Read the model definition and answer for the solid it produces. Units are mm, in the model's axes. A direction names the side the tool comes from. Coordinates: 2 decimals unless noted, no trailing zeros. Write each loop counter-clockwise with the first axis right and the second up, starting at its lowest first coordinate (ties: lowest second). Pieces come first, ordered by that corner, then holes. Notation, with made-up numbers: M 39.5,-35 L 66.5,-35 A10 ccw 66.5,-23 Z; hole C -4,-25.75 d8. An arc over 180 degrees is marked long. Write item = value, one per line.
from build123d import *

# Parameters (mm, degrees)
P_IDAT_VYSUNUT_M5_DEPTH = 1.6
P_IDAT_VYSUNUT_M6_DEPTH = 1
P_IDAT_VYSUNUT_M7_DEPTH = 3
ZKOSEN_1_SIZE           = 3
ZKOSEN_1_SIZE_2         = 1.398922974


with BuildPart() as part:
    # Skica1 → Přidat vysunutím5 (new body)
    with BuildSketch(Plane.XY):
        Polygon((0, 0), (0, 20), (-12.412784718, 31.615626352), (-23, 25), (-23, 0), align=None)
    extrude(amount=P_IDAT_VYSUNUT_M5_DEPTH)

    # Skica2 → Přidat vysunutím6 (add)
    with BuildSketch(Plane.XY.offset(1.6)):
        with BuildLine():
            Line((-3.705128205, 4.115384615), (-3.705128205, 2))
            Line((-3.705128205, 2), (-10.897435897, 2))
            add(Edge.make_bspline(
                [(-10.897435897, 2), (-10.87308441, 2.180790308), (-10.824395089, 2.542269551), (-10.673865117, 3.070299742), (-10.472959166, 3.585566992), (-10.254913916, 4.004869463), (-10.038043764, 4.342393523), (-9.841277463, 4.618963346), (-9.60654249, 4.913221767), (-9.337245105, 5.227544267), (-9.034873554, 5.562913411), (-8.697171951, 5.918082368), (-8.322529407, 6.291350846), (-8.058961705, 6.54481851), (-7.922676282, 6.67588141)],
                knots=[0, 0, 0, 0, 1.156289446, 2.311930546, 3.473459201, 4.661751613, 5.303057008, 6.018253237, 6.81459331, 7.690699809, 8.644447906, 9.679642995, 10.800191253, 12, 12, 12, 12], degree=3))
            add(Edge.make_bspline(
                [(-7.922676282, 6.67588141), (-7.813918956, 6.780862005), (-7.606877039, 6.980714138), (-7.312048947, 7.266894293), (-7.052864674, 7.529975199), (-6.823905036, 7.763139303), (-6.630459323, 7.972323552), (-6.469982936, 8.154242742), (-6.34044346, 8.309637702), (-6.270284768, 8.408220362), (-6.239182692, 8.451923077)],
                knots=[0, 0, 0, 0, 1.480720495, 2.818855715, 4.024636094, 5.098235712, 6.019786162, 6.815086302, 7.474715479, 8, 8, 8, 8], degree=3))
            add(Edge.make_bspline(
                [(-6.239182692, 8.451923077), (-6.175493233, 8.557718073), (-6.052643645, 8.761784362), (-5.91792888, 9.082682292), (-5.837068057, 9.403513936), (-5.825971765, 9.617891805), (-5.820512821, 9.723357372)],
                knots=[0, 0, 0, 0, 1.0911822, 2.104764037, 3.067617678, 4, 4, 4, 4], degree=3))
            add(Edge.make_bspline(
                [(-5.820512821, 9.723357372), (-5.824474653, 9.833108474), (-5.831970132, 10.040748999), (-5.894821019, 10.333768175), (-6.006276867, 10.585659667), (-6.15973106, 10.797196661), (-6.353774193, 10.962935085), (-6.580616259, 11.085399693), (-6.843577862, 11.153106661), (-7.028402789, 11.16201224), (-7.125, 11.166666667)],
                knots=[0, 0, 0, 0, 1.193122327, 2.257294386, 3.237245624, 4.168877528, 5.075331632, 5.990371598, 6.949684428, 8, 8, 8, 8], degree=3))
            add(Edge.make_bspline(
                [(-7.125, 11.166666667), (-7.220944609, 11.16231978), (-7.406288878, 11.153922533), (-7.669703299, 11.080565334), (-7.900142302, 10.953576306), (-8.06436539, 10.808860058), (-8.175305876, 10.668134018), (-8.250896853, 10.545500545), (-8.316050374, 10.406151312), (-8.37378183, 10.251655158), (-8.419383153, 10.080242168), (-8.456107626, 9.893217825), (-8.485702239, 9.689575671), (-8.495113848, 9.547907653), (-8.5, 9.474358974)],
                knots=[0, 0, 0, 0, 1.402788338, 2.709884207, 3.961032948, 5.225417836, 5.883680772, 6.578928686, 7.329201998, 8.132101139, 8.990263233, 9.922304639, 10.921339128, 12, 12, 12, 12], degree=3))
            Line((-8.5, 9.474358974), (-10.615384615, 9.681490385))
            add(Edge.make_bspline(
                [(-10.615384615, 9.681490385), (-10.598377251, 9.824305509), (-10.565402688, 10.101201217), (-10.483114114, 10.498918926), (-10.378898684, 10.865831465), (-10.247788098, 11.201257911), (-10.095201314, 11.507331251), (-9.913355139, 11.779458664), (-9.708603468, 12.020654551), (-9.480769352, 12.230790543), (-9.231301205, 12.410535137), (-8.969529148, 12.57098477), (-8.690337423, 12.702604473), (-8.396799939, 12.811078884), (-8.089049352, 12.897770766), (-7.765662274, 12.955090263), (-7.42863453, 12.995409017), (-7.198577984, 12.998446608), (-7.080929487, 13)],
                knots=[0, 0, 0, 0, 1.270971563, 2.464210789, 3.586263665, 4.638946707, 5.643716971, 6.603612468, 7.52484387, 8.434700188, 9.336036235, 10.239171475, 11.145359471, 12.059630629, 13.003312604, 13.96741569, 14.960557767, 16, 16, 16, 16], degree=3))
            add(Edge.make_bspline(
                [(-7.080929487, 13), (-6.953030371, 12.997541845), (-6.703930784, 12.992754281), (-6.34028961, 12.953218534), (-5.998674853, 12.884282231), (-5.676099879, 12.79296634), (-5.375877361, 12.67105295), (-5.095505554, 12.52366473), (-4.83939702, 12.345207999), (-4.603734114, 12.145414763), (-4.393070332, 11.925706984), (-4.20854792, 11.691351493), (-4.053955652, 11.442511564), (-3.924228998, 11.182220281), (-3.827907833, 10.90628918), (-3.757724044, 10.618533633), (-3.711189366, 10.317611197), (-3.707170936, 10.112088), (-3.705128205, 10.007612179)],
                knots=[0, 0, 0, 0, 1.210756838, 2.35810096, 3.457354827, 4.507168606, 5.527358126, 6.519769748, 7.499700793, 8.476517721, 9.440526811, 10.376769937, 11.295256217, 12.209626307, 13.124630862, 14.055668209, 15.011616881, 16, 16, 16, 16], degree=3))
            add(Edge.make_bspline(
                [(-3.705128205, 10.007612179), (-3.707819477, 9.887707131), (-3.713158546, 9.649833916), (-3.764276175, 9.298186238), (-3.84237396, 8.954647512), (-3.957796338, 8.618378159), (-4.104103161, 8.28131186), (-4.292696164, 7.942692037), (-4.511666905, 7.592306518), (-4.683112364, 7.36576699), (-4.771634615, 7.248798077)],
                knots=[0, 0, 0, 0, 0.953409949, 1.89141903, 2.821310783, 3.752688675, 4.715703262, 5.740811754, 6.833515735, 8, 8, 8, 8], degree=3))
            add(Edge.make_bspline(
                [(-4.771634615, 7.248798077), (-4.80509214, 7.206658226), (-4.876750403, 7.116404431), (-4.998659939, 6.978014195), (-5.139942605, 6.826848432), (-5.298602846, 6.660077667), (-5.479881522, 6.483607708), (-5.677256214, 6.290058721), (-5.899411985, 6.089331377), (-6.12951153, 5.876418507), (-6.360611244, 5.669193404), (-6.5730252, 5.472375498), (-6.765967752, 5.298233923), (-6.930453202, 5.137155265), (-7.076156545, 5.000133027), (-7.197826149, 4.880140867), (-7.29773874, 4.780083699), (-7.43541186, 4.624119958), (-7.610585282, 4.413178934), (-7.733826947, 4.21161882), (-7.792668269, 4.115384615)],
                knots=[0, 0, 0, 0, 0.665555651, 1.425465941, 2.280616993, 3.225313414, 4.272635571, 5.410053715, 6.644756443, 7.976022804, 9.288331007, 10.484517221, 11.558462543, 12.503158964, 13.33222979, 14.032602617, 14.617328242, 15.080653724, 16.606167857, 18, 18, 18, 18], degree=3))
            Line((-7.792668269, 4.115384615), (-3.705128205, 4.115384615))
        make_face()
    extrude(amount=P_IDAT_VYSUNUT_M6_DEPTH)

    # Skica3 → Přidat vysunutím7 (add)
    with BuildSketch(Plane.XY.offset(1.6)):
        Polygon((-15.200672089, 8.988396037), (-6.42438967, 19.447562139), (-11.786700772, 23.947075407), (-20.562983191, 13.487909304), align=None)
    extrude(amount=P_IDAT_VYSUNUT_M7_DEPTH)

    # Zkosení1
    # the kernel refuses this chamfer: 3, 1.398922974 mm, written as the material it takes off along each edge
    with BuildSketch(Plane(origin=(-26.517390277, 18.484250095, 4.6), x_dir=(-0.010484614203041273, -0.012495076643438774, -0.9998669641130704), z_dir=(0.7660444431189795, -0.6427876096865376, 0))) as zkosen_1_piece_1:
        Polygon((ZKOSEN_1_SIZE * 0.999866964113, ZKOSEN_1_SIZE * 0.0163111641311), (-ZKOSEN_1_SIZE_2 * 0.0163111641365, ZKOSEN_1_SIZE_2 * 0.999866964445), (0, 0), align=None)
    extrude(amount=14.772926414, mode=Mode.SUBTRACT)
    with BuildSketch(Plane(origin=(-6.790359982, 29.901482493, 4.6), x_dir=(-0.01249507664343894, 0.010484614203041415, -0.9998669641130704), z_dir=(-0.6427876096865377, -0.7660444431189796, 0)), Plane(origin=(-20.197012879, 3.03398895, 4.6), x_dir=(0.012495076643438493, -0.010484614203041037, -0.9998669641130704), z_dir=(0.6427876096865377, 0.7660444431189796, 0))) as zkosen_1_piece_2:
        Polygon((ZKOSEN_1_SIZE * 0.999866964113, ZKOSEN_1_SIZE * 0.0163111641311), (-ZKOSEN_1_SIZE_2 * 0.0163111641365, ZKOSEN_1_SIZE_2 * 0.999866964445), (0, 0), align=None)
    extrude(amount=29.199324499, mode=Mode.SUBTRACT)
    with BuildSketch(Plane(origin=(-0.469982584, 14.451221349, 4.6), x_dir=(0.010484614203041209, 0.01249507664343868, -0.9998669641130704), z_dir=(-0.766044443118979, 0.6427876096865381, 0))) as zkosen_1_piece_3:
        Polygon((ZKOSEN_1_SIZE * 0.999866964113, ZKOSEN_1_SIZE * 0.0163111641311), (-ZKOSEN_1_SIZE_2 * 0.0163111641365, ZKOSEN_1_SIZE_2 * 0.999866964445), (0, 0), align=None)
    extrude(amount=22.545852829, mode=Mode.SUBTRACT)


solid = part.part
Item 1: Find section C-C (x = -14.5). Determine the outline of the cut face in (y, z), and give its area (3 significant figures).
Worked answers:
outline = M 0,0 L 30.31,0 L 30.31,1.6 L 20.71,1.6 L 18.54,4.6 L 12,4.6 L 9.82,1.6 L 0,1.6 Z
area = 74.6 mm²
Item 2: Find section D-D (y = 27.5). Determine the outline of the cut face in (x, z).
Worked answers:
outline = M -19,0 L -8.01,0 L -8.01,1.6 L -19,1.6 Z
Item 3: Which of the six approach directions +Z, -Z, +X, -X, +Y, -Y give full straight-line access (tool end or side, diameter ignored) to faces 5 (the face through (-6, 8, 2.6)), 6 (the face through (-3.705, 3, 2)), 7 (the face through (-7, 2, 2)), 8 (the face through (-6, 4.115, 2))?
Worked answers:
face_5 = +Z, +X, -Y
face_6 = +Z, +X, +Y, -Y
face_7 = +Z, +X, -X, -Y
face_8 = +Z, +X
Item 4: Find section B-B (y = 20.5). Determine the outline of the cut face in (x, z).
Worked answers:
outline = M -23,0 L -0.53,0 L -0.53,1.6 L -7.68,1.6 L -9.85,4.6 L -12.85,4.6 L -14.68,1.6 L -23,1.6 Z
Item 5: Consider line 1 along Y through (x, z) = (-6, 1.95); line 2 along Z through (x, y) = (-7.25, 15.5); line 3 along Z through (x, y) = (-10.5, 10). Determine where each line is inside the solid, lowest interval first. Write a range as from..to.
Worked answers:
line_1 = 2..4.12, 6..8.89, 10.56..12.88
line_2 = 0..1.6
line_3 = 0..2.6
Item 6: Find section A-A (z = 0.9). Determine the outline of the cut face in (x, y).
Worked answers:
outline = M -23,0 L 0,0 L 0,20 L -12.41,31.62 L -23,25 Z
Item 7: For a pull along X with two mould halves and no side action, classify faces 1 (the face through (-9.543, 9.576, 2.093)), 2 (the face through (-12, 0, 1)), 3 (the face through (-11.4, 14.59, 3.08)), 4 (the face through (-9.511, 21.138, 3.079)) as released by +X, released by -X, zero draft, split by the parting line, or undercut.
Worked answers:
face_1 = undercut
face_2 = zero draft
face_3 = undercut
face_4 = released by +X
Item 8: A flat-ended cylindrical pin translates along its axis: pin 1 (6 mm diameter, centred on x = -8.5, y = 6, fed in from +Z). Find the tip coordinate at first contact, or state that the pin passes through.
Worked answers:
pin_1 = 2.6
